```python
from build123d import *

# Parameters (mm, degrees)
SKETCH_1_W                       = 45
SKETCH_1_H                       = 20
EXTRUDE_1_DEPTH                  = 0.5
SM_EDGE_FLANGE_1_STRIP_W         = 3
SM_EDGE_FLANGE_1_STRIP_H         = 0.5
SM_EDGE_FLANGE_1_STRIP_CUT_DEPTH = 45
SM_EDGE_FLANGE_1_DEPTH           = 45
SKETCH_9_R                       = 2
CUT_EXTRUDE_1_DEPTH              = 0.5
CUT_EXTRUDE_2_DEPTH              = 0.5
SKETCH_11_R                      = 1.5
CUT_EXTRUDE_3_DEPTH              = 0.5
FILLET_1_R                       = 3
FILLET_2_R                       = 2


# Sheet-metal steps are written as plain solids
with BuildPart() as part:
    # Sketch 1 → Бобышка-Вытянуть1 (new body)
    with BuildSketch(Plane(origin=(0, 0, 0), x_dir=(1, 0, 0), z_dir=(0, 1, 0))):
        Rectangle(SKETCH_1_W, SKETCH_1_H)
    extrude(amount=EXTRUDE_1_DEPTH)

    # Ребро-кромка1 strip (across the edge) → Ребро-кромка1 strip cut (cut)
    with BuildSketch(Plane(origin=(-22.5, 0.5, 10), x_dir=(0, 0, -1), z_dir=(1, 0, 0))):
        with Locations((-0.5, -0.25)):
            Rectangle(SM_EDGE_FLANGE_1_STRIP_W, SM_EDGE_FLANGE_1_STRIP_H)
    extrude(amount=SM_EDGE_FLANGE_1_STRIP_CUT_DEPTH, mode=Mode.SUBTRACT)

    # Ребро-кромка1 section (across the edge) → Ребро-кромка1 (add)
    with BuildSketch(Plane(origin=(-22.5, 0.5, 10), x_dir=(0, 0, -1), z_dir=(1, 0, 0))):
        with BuildLine():
            Line((0, 0.5), (0, 20.5))
            Line((0, 20.5), (0.5, 20.5))
            Line((0.5, 20.5), (0.5, 0.5))
            ThreePointArc((0.5, 0.5), (0.646446609, 0.146446609), (1, 0))
            Line((1, 0), (1, -0.5))
            ThreePointArc((1, -0.5), (0.292893219, -0.207106781), (0, 0.5))
        make_face()
    extrude(amount=SM_EDGE_FLANGE_1_DEPTH)

    # Эскиз9 → Вырез-Вытянуть1 (cut)
    with BuildSketch(Plane.XY.offset(10)):
        with Locations((-17.5, 17.5)):
            Circle(SKETCH_9_R)
        with Locations(Location((17.5, 17.5, 0), (0, 0, 180))):
            Circle(SKETCH_9_R)
    extrude(amount=-CUT_EXTRUDE_1_DEPTH, mode=Mode.SUBTRACT)

    # Эскиз10 → Вырез-Вытянуть2 (cut)
    with BuildSketch(Plane(origin=(0, 0.5, 0), x_dir=(1, 0, 0), z_dir=(0, 1, 0))):
        with BuildLine():
            Line((-5.5, -4), (5.5, -4))
            ThreePointArc((5.5, -4), (8, -6.5), (5.5, -9))
            Line((5.5, -9), (-5.5, -9))
            ThreePointArc((-5.5, -9), (-8, -6.5), (-5.5, -4))
        make_face()
    extrude(amount=-CUT_EXTRUDE_2_DEPTH, mode=Mode.SUBTRACT)

    # Эскиз11 → Вырез-Вытянуть3 (cut)
    with BuildSketch(Plane(origin=(0, 0.5, 0), x_dir=(1, 0, 0), z_dir=(0, 1, 0))):
        with Locations(Location((-16.5, 2, 0), (0, 0, 270))):
            Circle(SKETCH_11_R)
        with Locations(Location((16.5, 2, 0), (0, 0, 90))):
            Circle(SKETCH_11_R)
    extrude(amount=-CUT_EXTRUDE_3_DEPTH, mode=Mode.SUBTRACT)

    # Скругление1
    fillet_1_edges = [part.edges().sort_by_distance(p)[0] for p in [
        (-22.5, 21, 9.75),
        (22.5, 21, 9.75),
    ]]
    fillet(fillet_1_edges, radius=FILLET_1_R)

    # Скругление2
    fillet_2_edges = [part.edges().sort_by_distance(p)[0] for p in [
        (22.5, 0.25, -10),
        (-22.5, 0.25, -10),
    ]]
    fillet(fillet_2_edges, radius=FILLET_2_R)


solid = part.part
```
The listing builds one solid part. Answer for the finished solid, in the listing's coordinates (mm). A direction names the side the tool comes from. Coordinates: 2 decimals unless noted, no trailing zeros. Write each loop counter-clockwise with the first axis right and the second up, starting at its lowest first coordinate (ties: lowest second). Pieces come first, ordered by that corner, then holes. Notation, with made-up numbers: M 76,13.25 L 115,13.25 A25 ccw 115,43.25 Z; hole C 59,-39 d3. An arc over 180 degrees is marked long. Use a Markdown table: item, result. Add a question column.
1. Straight lines are drawn through the part: line 1 along X through (y, z) = (0.25, -2); line 2 along Z through (x, y) = (17, 7); line 3 along Y through (x, z) = (12, -1). For each, find the intervals that lie inside material, in ascending order. Write a range as [from, to].
2. Section D-D (x = -17.5) is taken. Give the vertices of the cut face in (y, z), plus the area to 3 significant figures.
3. Section B-B (z = 6.5) is taken. Give the vertices of the cut face in (x, y).
4. Which of the six approach directions +Z, -Z, +X, -X, +Y, -Y give full straight-line access (tool end or side, diameter ignored) to faces 1 (the flat face through (0, 0, -1)), 2 (the cylindrical face through (-8, 0.3, 6.6)), 3 (the flat face through (0, 11, 9.5))?
5. Section A-A (x = 4) is taken. Give the vertices of the cut face in (y, z), plus the area to 3 significant figures.
6. For a pull along Z with two mould halves and no side action, classify faces 4 (the cylindrical face through (-21.64, 20.1, 9.75)), 5 (the cylindrical face through (16.43, 0.25, -0.5)), 6 (the cylindrical face through (-0.315, 0.285, 9.699)), 7 (the cylindrical face through (21.93, 0.25, -9.4)) as +Z half, -Z half, draft (parallel to the pull), parting line (faces both ways), or undercut.
7. Section C-C (x = 13) is taken. Give the vertices of the cut face in (y, z).
8. Given P1, Ø1.8, axis at x = 16.5, z = -2, coming from the +Y side; P2, Ø2, axis at x = -6, y = 3.5, coming from the -Z side; P3, Ø9.5, axis at x = -2.5, z = -5, coming from the +Y side, each flat-ended and moving along its own axis, determine where each tip first touches the part or whether it passes through.
Data:
| question | item | result |
|---|---|---|
| 1 | line 1 | x = [-22.5, -18], [-15, 15], [18, 22.5] |
| 1 | line 2 | z = [9.5, 10] |
| 1 | line 3 | y = [0, 0.5] |
| 2 | outline | M 0,-10 L 0.5,-10 L 0.5,-3.12 L 0,-3.12 Z; M 0,-0.88 L 0.5,-0.88 L 0.5,9 A0.5 cw 1,9.5 L 15.5,9.5 L 15.5,10 L 1,10 A1 ccw 0,9 Z; M 19.5,9.5 L 21,9.5 L 21,10 L 19.5,10 Z |
| 2 | area | 17.0 mm2 |
| 3 | outline | M -22.5,0 L -8,0 L -8,0.5 L -22.5,0.5 Z; M 8,0 L 22.5,0 L 22.5,0.5 L 8,0.5 Z |
| 4 | face 1 | +Z, -Z, +X, -X, -Y |
| 4 | face 2 | +Y, -Y |
| 4 | face 3 | -Z, +X, -X, +Y |
| 5 | outline | M 0,-10 L 0.5,-10 L 0.5,4 L 0,4 Z; M 0,9 L 0.5,9 A0.5 cw 1,9.5 L 21,9.5 L 21,10 L 1,10 A1 ccw Z |
| 5 | area | 17.6 mm2 |
| 6 | face 4 | draft |
| 6 | face 5 | undercut |
| 6 | face 6 | +Z half |
| 6 | face 7 | -Z half |
| 7 | outline | M 0,-10 L 0.5,-10 L 0.5,9 A0.5 cw 1,9.5 L 21,9.5 L 21,10 L 1,10 A1 ccw 0,9 Z |
| 8 | P1 | passes through |
| 8 | P2 | stops at z = 9.5 |
| 8 | P3 | stops at y = 0.5 |
